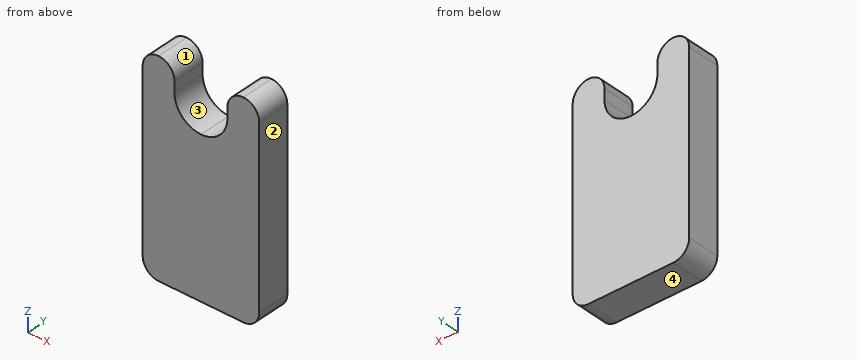
```python
from build123d import *

# Parameters (mm, degrees)
BOSS_EXTRUDE1_DEPTH = 3.08
FILLET1_R           = 2.5
FILLET2_R           = 1.5


with BuildPart() as part:
    # Sketch2 → Boss-Extrude1 (new body)
    with BuildSketch(Plane(origin=(0, 0, 0), x_dir=(1, 0, 0), z_dir=(0, 1, 0))):
        Polygon((-2.5, 2.5), (-2.5, -2.5), (-5.5, -2.5), (-5.5, 17), (5.5, 17), (5.5, -2.5), (2.5, -2.5), (2.5, 2.5), align=None)
    extrude(amount=BOSS_EXTRUDE1_DEPTH)

    # Fillet1
    fillet1_edges = [part.edges().sort_by_distance(p)[0] for p in [
        (-2.5, 1.54, -2.5),
        (2.5, 1.54, -2.5),
    ]]
    fillet(fillet1_edges, radius=FILLET1_R - 0.0001)  # a hair under: the kernel refuses the full size

    # Fillet2
    fillet2_edges = [part.edges().sort_by_distance(p)[0] for p in [
        (-5.5, 1.54, -17),
        (5.5, 1.54, -17),
        (5.5, 1.54, 2.5),
        (2.5, 1.54, 2.5),
        (-5.5, 1.54, 2.5),
        (-2.5, 1.54, 2.5),
    ]]
    fillet(fillet2_edges, radius=FILLET2_R - 0.0001)  # a hair under: the kernel refuses the full size


solid = part.part
```
Input: part model. Units: mm. Frame: model coordinates. Face numbers are marked on the shaded views. Round coordinates to 2 decimals unless told otherwise and drop trailing zeros. Write each loop counter-clockwise with the first axis right and the second up, starting at its lowest first coordinate (ties: lowest second). Pieces come first, ordered by that corner, then holes. Notation, with made-up numbers: M -38,25 L 1,25 A28 cw 1,43 Z; hole C 74.5,43 d4. An arc over 180 degrees is marked long. Write each question's results on one line, items separated by ' | '.
Q1. Section query C-C (z = 1.25). Return loops of the section in (x, y).
Results:
outline: M -5.48,0 L -2.52,0 L -2.52,3.08 L -5.48,3.08 Z; M 2.52,0 L 5.48,0 L 5.48,3.08 L 2.52,3.08 Z
Q2. Draft query along X for the marked faces 1, 2, 3 and 4. Return one class per face: released by +X, released by -X, zero draft, split by the parting line, or undercut.
Results:
face 1: undercut | face 2: released by +X | face 3: undercut | face 4: zero draft
Q3. Line query: line 1 along X through (y, z) = (2.55, -2); line 2 along X through (y, z) = (0.95, -0.75); line 3 along Z through (x, y) = (-2, 0.85). Output: solid intervals per line, ascending.
Results:
line 1: x = -5.5 to -1.5, 1.5 to 5.5 | line 2: x = -5.5 to -2.38, 2.38 to 5.5 | line 3: z = -17 to -1.5
Q4. Section query A-A (z = -2.25). Return loops of the section in (x, y).
Results:
outline: M -5.5,0 L -1.09,0 L -1.09,3.08 L -5.5,3.08 Z; M 1.09,0 L 5.5,0 L 5.5,3.08 L 1.09,3.08 Z
